Check sheet for the modelled part. Datum: model origin and axes. Units: mm. A direction names the side the tool comes from. Coordinates: 2 decimals unless noted, no trailing zeros. Write each loop counter-clockwise with the first axis right and the second up, starting at its lowest first coordinate (ties: lowest second). Pieces come first, ordered by that corner, then holes. Notation, with made-up numbers: (-23, -8) -> (-19, -8) arc R10 ccw to (-19, 10) -> close; hole circle Ø4 at (82, 78). An arc over 180 degrees is marked (long way). Put each result on its own line as item: value.
```python
from build123d import *

# Parameters (mm, degrees)
F1_DEPTH       = 8.15
F1_TAPER       = 20
F2_T           = -4
F4_DEPTH       = 5
F4_TAPER       = 23
F6_D           = 6.35
F6_CBORE_D     = 11
F6_CBORE_DEPTH = 2.5


with BuildPart() as f1:
    # F0 (on Top) → F1 (new body)
    with BuildSketch(Plane.XY):
        with BuildLine():
            ThreePointArc((13.5235004185, 24.6379186874), (12.605417789, 25.1846935831), (11.5539321881, 25.375))
            Line((11.5539321881, 25.375), (-12.9567069347, 25.375))
            ThreePointArc((-12.9567069347, 25.375), (-14.1999477217, 25.1052659844), (-15.2196256222, 24.3445682304))
            Line((-15.2196256222, 24.3445682304), (-24.6379186874, 13.5235004185))
            ThreePointArc((-24.6379186874, 13.5235004185), (-25.1846935831, 12.605417789), (-25.375, 11.5539321881))
            Line((-25.375, 11.5539321881), (-25.375, -12.6529412227))
            ThreePointArc((-25.375, -12.6529412227), (-25.1255957189, -13.8505318001), (-24.4188512059, -14.8489995662))
            Line((-24.4188512059, -14.8489995662), (-13.972783394, -24.5710583435))
            ThreePointArc((-13.972783394, -24.5710583435), (-13.0270726549, -25.1667893035), (-11.9289321881, -25.375))
            Line((-11.9289321881, -25.375), (11.9289321881, -25.375))
            ThreePointArc((11.9289321881, -25.375), (13.0270726549, -25.1667893035), (13.972783394, -24.5710583435))
            Line((13.972783394, -24.5710583435), (24.4188512059, -14.8489995662))
            ThreePointArc((24.4188512059, -14.8489995662), (25.1255957189, -13.8505318001), (25.375, -12.6529412227))
            Line((25.375, -12.6529412227), (25.375, 12.9567069347))
            ThreePointArc((25.375, 12.9567069347), (25.1052659844, 14.1999477217), (24.3445682304, 15.2196256222))
            Line((24.3445682304, 15.2196256222), (13.5235004185, 24.6379186874))
        make_face()
    extrude(amount=F1_DEPTH, taper=F1_TAPER)

    # F2
    f2_openings = [f1.faces().sort_by_distance(p)[0] for p in [
        (0.016382, 0.006023, 0),
    ]]
    offset(amount=F2_T, openings=f2_openings)

    # F3 (on face) → F4 (join)
    with BuildSketch(Plane.XY.offset(8.15)):
        with BuildLine():
            ThreePointArc((35, 22.5), (33.5355339059, 26.0355339059), (30, 27.5))
            Line((30, 27.5), (-30, 27.5))
            ThreePointArc((-30, 27.5), (-33.5355339059, 26.0355339059), (-35, 22.5))
            Line((-35, 22.5), (-35, -22.5))
            ThreePointArc((-35, -22.5), (-33.5355339059, -26.0355339059), (-30, -27.5))
            Line((-30, -27.5), (30, -27.5))
            ThreePointArc((30, -27.5), (33.5355339059, -26.0355339059), (35, -22.5))
            Line((35, -22.5), (35, 22.5))
        make_face()
        with BuildLine():
            Line((11.5760193141, 22.4003768158), (22.397087126, 12.9820837505))
            ThreePointArc((22.397087126, 12.9820837505), (22.4056177404, 12.9706488817), (22.4086425907, 12.9567069347))
            Line((22.4086425907, 12.9567069347), (22.4086425907, -12.6529412227))
            ThreePointArc((22.4086425907, -12.6529412227), (22.405845722, -12.6663712392), (22.3979201499, -12.6775682533))
            Line((22.3979201499, -12.6775682533), (11.951852338, -22.3996270307))
            ThreePointArc((11.951852338, -22.3996270307), (11.9412469516, -22.406307675), (11.9289321881, -22.4086425907))
            Line((11.9289321881, -22.4086425907), (-11.9289321881, -22.4086425907))
            ThreePointArc((-11.9289321881, -22.4086425907), (-11.9412469516, -22.406307675), (-11.951852338, -22.3996270307))
            Line((-11.951852338, -22.3996270307), (-22.3979201499, -12.6775682533))
            ThreePointArc((-22.3979201499, -12.6775682533), (-22.405845722, -12.6663712392), (-22.4086425907, -12.6529412227))
            Line((-22.4086425907, -12.6529412227), (-22.4086425907, 11.5539321881))
            ThreePointArc((-22.4086425907, 11.5539321881), (-22.4065084571, 11.5657237547), (-22.4003768158, 11.5760193141))
            Line((-22.4003768158, 11.5760193141), (-12.9820837505, 22.397087126))
            ThreePointArc((-12.9820837505, 22.397087126), (-12.9706488817, 22.4056177404), (-12.9567069347, 22.4086425907))
            Line((-12.9567069347, 22.4086425907), (11.5539321881, 22.4086425907))
            ThreePointArc((11.5539321881, 22.4086425907), (11.5657237547, 22.4065084571), (11.5760193141, 22.4003768158))
        make_face(mode=Mode.SUBTRACT)
        with BuildLine():
            ThreePointArc((22.4086425907, 12.9567069347), (22.4056177404, 12.9706488817), (22.397087126, 12.9820837505))
            Line((22.397087126, 12.9820837505), (11.5760193141, 22.4003768158))
            ThreePointArc((11.5760193141, 22.4003768158), (11.5657237547, 22.4065084571), (11.5539321881, 22.4086425907))
            Line((11.5539321881, 22.4086425907), (-12.9567069347, 22.4086425907))
            ThreePointArc((-12.9567069347, 22.4086425907), (-12.9706488817, 22.4056177404), (-12.9820837505, 22.397087126))
            Line((-12.9820837505, 22.397087126), (-22.4003768158, 11.5760193141))
            ThreePointArc((-22.4003768158, 11.5760193141), (-22.4065084571, 11.5657237547), (-22.4086425907, 11.5539321881))
            Line((-22.4086425907, 11.5539321881), (-22.4086425907, -12.6529412227))
            ThreePointArc((-22.4086425907, -12.6529412227), (-22.405845722, -12.6663712392), (-22.3979201499, -12.6775682533))
            Line((-22.3979201499, -12.6775682533), (-11.951852338, -22.3996270307))
            ThreePointArc((-11.951852338, -22.3996270307), (-11.9412469516, -22.406307675), (-11.9289321881, -22.4086425907))
            Line((-11.9289321881, -22.4086425907), (11.9289321881, -22.4086425907))
            ThreePointArc((11.9289321881, -22.4086425907), (11.9412469516, -22.406307675), (11.951852338, -22.3996270307))
            Line((11.951852338, -22.3996270307), (22.3979201499, -12.6775682533))
            ThreePointArc((22.3979201499, -12.6775682533), (22.405845722, -12.6663712392), (22.4086425907, -12.6529412227))
            Line((22.4086425907, -12.6529412227), (22.4086425907, 12.9567069347))
        make_face()
    extrude(amount=F4_DEPTH, taper=F4_TAPER)

    # F6 (through all)
    with Locations(Plane.XY.offset(13.15)):
        with Locations((0, 0)):
            CounterBoreHole(F6_D / 2, F6_CBORE_D / 2, F6_CBORE_DEPTH)


solid = f1.part
```
Q1. Cross-section at B-B (y = 0). Record the cut outline in (x, z) (3 decimals).
Recorded:
outline: (-35, 8.15) -> (-22.409, 8.15) -> (-25.375, 0) -> (-21.118, 0) -> (-19.608, 4.15) -> (-3.175, 4.15) -> (-3.175, 10.65) -> (-5.5, 10.65) -> (-5.5, 13.15) -> (-32.878, 13.15) -> close; (3.175, 4.15) -> (19.608, 4.15) -> (21.118, 0) -> (25.375, 0) -> (22.409, 8.15) -> (35, 8.15) -> (32.878, 13.15) -> (5.5, 13.15) -> (5.5, 10.65) -> (3.175, 10.65) -> close
Q2. Cross-section at D-D (y = -18). Record the cut outline in (x, z), plus the area to 3 significant figures.
Recorded:
outline: (-35, 8.15) -> (-16.68, 8.15) -> (-21.03, 0) -> (-14.79, 0) -> (-12.57, 4.15) -> (12.57, 4.15) -> (14.79, 0) -> (21.03, 0) -> (16.68, 8.15) -> (35, 8.15) -> (32.88, 13.15) -> (-32.88, 13.15) -> close
area: 533 mm2
Q3. Mould release check, pull along X, two halves, no side actions. Record for faces 1 (the flat face through (-0.815, 20.374, 2.046)), 2 (the flat face through (-23.91, -0.72, 4.02)), 3 (the flat face through (23.91, 0.33, 4.02)): released by +X, released by -X, zero draft, split by the parting line, or undercut.
Recorded:
face 1: undercut
face 2: released by -X
face 3: released by +X
Q4. Depth check by flat-ended pin: P1, Ø3, axis at x = -21, z = 4.5, coming from the -Y side; P2, Ø2, axis at x = -14.5, z = 5, coming from the -Y side; P3, Ø1.5, axis at x = 20.5, z = 1.5, coming from the +Y side. Enter the tip coordinate at first touch or a pass-through.
Recorded:
P1: stops at y = -17.38
P2: stops at y = -22.65
P3: stops at y = 18.59
Q5. Material ranges on line 1 along Z through (x, y) = (0, -5); line 2 along Z through (x, y) = (27, 20); line 3 along X through (y, z) = (-13, 1), recorded low to high.
Recorded:
line 1: z = 4.15 to 10.65
line 2: z = 8.15 to 13.15
line 3: x = -24.99 to -19.62, 19.62 to 24.99
Q6. Cross-section at A-A (x = 0). Record the cut outline in (y, z) (3 decimals), plus the area to 3 significant figures.
Recorded:
outline: (-27.5, 8.15) -> (-22.409, 8.15) -> (-25.375, 0) -> (-21.118, 0) -> (-19.608, 4.15) -> (-3.175, 4.15) -> (-3.175, 10.65) -> (-5.5, 10.65) -> (-5.5, 13.15) -> (-25.378, 13.15) -> close; (3.175, 4.15) -> (19.608, 4.15) -> (21.118, 0) -> (25.375, 0) -> (22.409, 8.15) -> (27.5, 8.15) -> (25.378, 13.15) -> (5.5, 13.15) -> (5.5, 10.65) -> (3.175, 10.65) -> close
area: 416 mm2
Q7. Tool access check on faces 4 (the flat face through (0, -4, 4.15)), 5 (the conical face through (-12.484, -23.764, 4.132)), 6 (the flat face through (18.27, -18.57, 4.02)), 7 (the flat face through (0.17, -23.91, 4.02)), 8 (the conical face through (23.74, 13.57, 4.13)). Record the directions out of +Z, -Z, +X, -X, +Y, -Y that give a thin tool (end or side, any length) a straight path to the whole face; none if there is none.
Recorded:
face 4: -Z
face 5: -X, -Y
face 6: +X, -Y
face 7: +X, -X, -Y
face 8: +X, +Y
Q8. Cross-section at C-C (z = 6). Record the cut outline in (x, y) (3 decimals).
Recorded:
outline: (-23.191, -12.653) arc R0.816 ccw to (-22.931, -13.25) -> (-12.485, -22.972) arc R0.816 ccw to (-11.929, -23.191) -> (11.929, -23.191) arc R0.816 ccw to (12.485, -22.972) -> (22.931, -13.25) arc R0.816 ccw to (23.191, -12.653) -> (23.191, 12.957) arc R0.816 ccw to (22.911, 13.572) -> (12.09, 22.991) arc R0.816 ccw to (11.554, 23.191) -> (-12.957, 23.191) arc R0.816 ccw to (-13.572, 22.911) -> (-22.991, 12.09) arc R0.816 ccw to (-23.191, 11.554) -> close; hole circle Ø6.35 at (0, 0)
